```python
from build123d import *

# Parameters (mm, degrees)
SKETCH1_R             = 2
BOSS_EXTRUDE1_DEPTH   = 4
SKETCH2_R             = 2.5
BOSS_EXTRUDE2_DEPTH   = 17
CUT_EXTRUDE1_START    = -17
CUT_EXTRUDE1_DEPTH    = 17
SKETCH4_R             = 2
BOSS_EXTRUDE3_DEPTH   = 11
BODY_MOVE_COPY3_ANGLE = 90
BODY_MOVE_COPY5_ANGLE = 90
CUT_EXTRUDE2_START    = -10
CUT_EXTRUDE2_DEPTH    = 10


with BuildPart() as part:
    # Sketch1 → Boss-Extrude1 (new body)
    with BuildSketch(Plane(origin=(0, 0, 0), x_dir=(1, 0, 0), z_dir=(0, 1, 0))):
        with Locations(Location((0, 0, 0), (0, 0, 270))):
            Circle(SKETCH1_R)
    extrude(amount=BOSS_EXTRUDE1_DEPTH)

    # Sketch2 → Boss-Extrude2 (add)
    with BuildSketch(Plane(origin=(0, 4, 0), x_dir=(1, 0, 0), z_dir=(0, 1, 0))):
        with Locations(Location((0, 0, 0), (0, 0, 270))):
            Circle(SKETCH2_R)
    extrude(amount=BOSS_EXTRUDE2_DEPTH)

    # Sketch3 → Cut-Extrude1 (cut)
    with BuildSketch(Plane(origin=(0, 21, 0), x_dir=(1, 0, 0), z_dir=(0, 1, 0)).offset(CUT_EXTRUDE1_START)):
        with BuildLine():
            Line((1.5, 2), (-1.5, 2))
            ThreePointArc((-1.5, 2), (0, 2.5), (1.5, 2))
        make_face()
    extrude(amount=CUT_EXTRUDE1_DEPTH, mode=Mode.SUBTRACT)

    # Sketch4 → Boss-Extrude3 (add)
    with BuildSketch(Plane(origin=(0, 21, 0), x_dir=(1, 0, 0), z_dir=(0, 1, 0))):
        with Locations(Location((0, 0, 0), (0, 0, 90))):
            Circle(SKETCH4_R)
    extrude(amount=BOSS_EXTRUDE3_DEPTH)


with BuildPart() as part_1:
    # Body-Move/Copy3: moved
    add(part.part.rotate(Axis((0, 15.5, 0), (0, 0, 1)), BODY_MOVE_COPY3_ANGLE))


with BuildPart() as part_2:
    # Body-Move/Copy5: moved
    add(part_1.part.rotate(Axis((0, 15.5, 0.25), (1, 0, 0)), BODY_MOVE_COPY5_ANGLE))

    # Sketch5 → Cut-Extrude2 (cut)
    with BuildSketch(Plane.ZY.offset(16.5).offset(CUT_EXTRUDE2_START)):
        with BuildLine():
            Line((-1.072875656, 17.25), (1.572875656, 17.25))
            ThreePointArc((1.572875656, 17.25), (0.25, 17.75), (-1.072875656, 17.25))
        make_face()
    extrude(amount=CUT_EXTRUDE2_DEPTH, mode=Mode.SUBTRACT)


solid = part_2.part
```
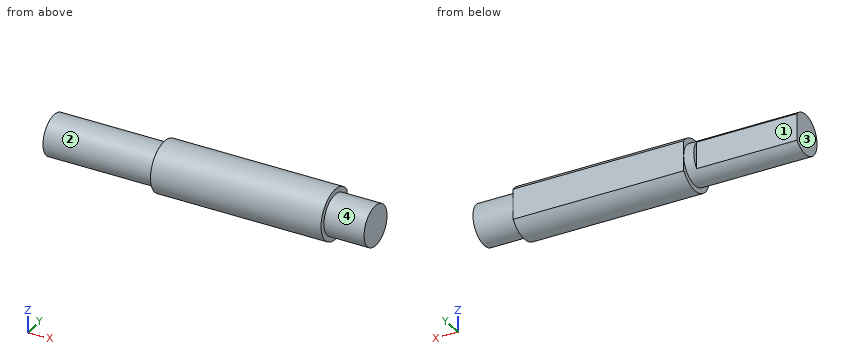
The listing builds one solid part. Answer for the finished solid, in the listing's coordinates (mm). Face numbers are marked on the shaded views. A direction names the side the tool comes from. Round coordinates to 2 decimals unless told otherwise and drop trailing zeros. Write each loop counter-clockwise with the first axis right and the second up, starting at its lowest first coordinate (ties: lowest second). Pieces come first, ordered by that corner, then holes. Notation, with made-up numbers: (10, 46) -> (48, 46) arc R21 ccw to (48, 82) -> close; hole circle Ø5 at (67.25, 73.5). An arc over 180 degrees is marked (long way). Answer as a JSON object with one key per item and string values. Group by question number.
Q1. Each of these flat-tipped pins is pushed along its axis until it touches: pin 1 Ø3 at (x, z) = (12, -0.5) entering from +Y; pin 2 Ø2 at (x, z) = (-11.5, 0) entering from +Y. Where does it stop, or does it pass through?
Q2. Section D-D (y = 16.9) is taken. Write down the section's boundary in (x, z).
Q3. Section A-A (y = 15.75) is taken. Write down the section's boundary in (x, z).
Q4. Section B-B (x = -6) is taken. Write down the section's boundary in (y, z).
Q5. Straight lines are drawn through the part: line 1 along X through (y, z) = (17.4, 0.6); line 2 along X through (y, z) = (14.95, 2.45); line 3 along Z through (x, y) = (-10.5, 15.6). For each, find the intervals that lie inside material, in ascending order.
Q6. Which of the six approach directions +Z, -Z, +X, -X, +Y, -Y give full straight-line access (tool end or side, diameter ignored) to the marked faces 1, 2, 3 and 4?
Check values:
{
 "1": {"pin 1": "y = 17.75", "pin 2": "y = 17.25"},
 "2": {"outline": "(-16.5, -1.39) -> (-5.5, -1.39) -> (-5.5, -1.97) -> (11.5, -1.97) -> (11.5, -1.39) -> (15.5, -1.39) -> (15.5, 1.89) -> (11.5, 1.89) -> (11.5, 2.47) -> (-5.5, 2.47) -> (-5.5, 1.89) -> (-16.5, 1.89) -> close"},
 "3": {"outline": "(-16.5, -1.75) -> (-5.5, -1.75) -> (-5.5, -2.25) -> (11.5, -2.25) -> (11.5, -1.75) -> (15.5, -1.75) -> (15.5, 2.25) -> (11.5, 2.25) -> (11.5, 2.75) -> (-5.5, 2.75) -> (-5.5, 2.25) -> (-16.5, 2.25) -> close"},
 "4": {"outline": "circle Ø4 at (15.75, 0.25)"},
 "5": {"line 1": "-6.5 to 15.5", "line 2": "-5.5 to 11.5", "line 3": "-1.74 to 2.24"},
 "6": {"face 1": "+Z, -Z, -X, +Y", "face 2": "-X", "face 3": "+Z, -Z, -X, +Y, -Y", "face 4": "+X"}
}
